```python
from build123d import *

# Parameters (mm, degrees)
F0_W      = 165
F0_H      = 45
F0_R      = 12.5
F1_DEPTH  = 1
F3_DEPTH  = 1
F4_DEPTH  = 25
F5_DEPTH  = 25
F8_DEPTH  = 1
F9_W      = 35.9933748841
F9_H      = 31.3726086169
F9_W_2    = 33.6829945445
F9_H_2    = 28.8190245628
F10_DEPTH = 1
F11_R     = 4.1249872097
F12_DEPTH = 25
F13_R     = 2.1502393586
F14_DEPTH = 25
F15_R     = 5
F16_DEPTH = 25


with BuildPart() as f1:
    # F0 (on Front) → F1 (new body)
    with BuildSketch(Plane.XZ):
        Rectangle(F0_W, F0_H)
        with Locations((-65, 0)):
            Circle(F0_R, mode=Mode.SUBTRACT)
        with Locations((65, 0)):
            Circle(F0_R, mode=Mode.SUBTRACT)
    extrude(amount=F1_DEPTH)

    # F2 (on face) → F3 (join)
    with BuildSketch(Plane.XZ.offset(1)):
        with BuildLine():
            Line((68.3925151825, -19.0988145769), (65, -22.5))
            ThreePointArc((65, -22.5), (87.5, 0), (65, 22.5))
            Line((65, 22.5), (71.474224329, 16.2770561874))
            Line((71.474224329, 16.2770561874), (77.4062722921, 9.1145541519))
            Line((77.4062722921, 9.1145541519), (80.3926512599, 2.1407562308))
            Line((80.3926512599, 2.1407562308), (80.3926512599, -5.2317115478))
            Line((80.3926512599, -5.2317115478), (78.3914923668, -12.1520543471))
            Line((78.3914923668, -12.1520543471), (74.6632069349, -14.4081749022))
            Line((74.6632069349, -14.4081749022), (68.3925151825, -19.0988145769))
        make_face()
        with BuildLine():
            Line((-65, 14.9617949501), (-65, 22.5))
            ThreePointArc((-65, 22.5), (-87.5, 0), (-65, -22.5))
            Line((-65, -22.5), (-67.4760043621, -15.6979020685))
            Line((-67.4760043621, -15.6979020685), (-72.8440880775, -12.9142012447))
            Line((-72.8440880775, -12.9142012447), (-76.5851810575, -7.8018400818))
            Line((-76.5851810575, -7.8018400818), (-79.5639529824, 0))
            Line((-79.5639529824, 0), (-79.5639529824, 6.4657721668))
            Line((-79.5639529824, 6.4657721668), (-75.4495188594, 11.7608513683))
            Line((-75.4495188594, 11.7608513683), (-65, 14.9617949501))
        make_face()
    extrude(amount=-F3_DEPTH)

    # F2 (on face) → F4 (cut)
    with BuildSketch(Plane.XZ.offset(1)):
        with BuildLine():
            Line((-82.5, 22.5), (-82.5, 14.1421356237))
            ThreePointArc((-82.5, 14.1421356237), (-74.6966991411, 20.3033008589), (-65, 22.5))
            Line((-65, 22.5), (-82.5, 22.5))
        make_face()
    extrude(amount=-F4_DEPTH, mode=Mode.SUBTRACT)

    # F2 (on face) → F5 (cut)
    with BuildSketch(Plane.XZ.offset(1)):
        with BuildLine():
            ThreePointArc((82.5, -14.1421356237), (74.6966991411, -20.3033008589), (65, -22.5))
            Line((65, -22.5), (82.5, -22.5))
            Line((82.5, -22.5), (82.5, -14.1421356237))
        make_face()
        with BuildLine():
            ThreePointArc((65, 22.5), (74.6966991411, 20.3033008589), (82.5, 14.1421356237))
            Line((82.5, 14.1421356237), (82.5, 22.5))
            Line((82.5, 22.5), (65, 22.5))
        make_face()
        with BuildLine():
            Line((-82.5, -22.5), (-65, -22.5))
            ThreePointArc((-65, -22.5), (-74.6966991411, -20.3033008589), (-82.5, -14.1421356237))
            Line((-82.5, -14.1421356237), (-82.5, -22.5))
        make_face()
    extrude(amount=-F5_DEPTH, mode=Mode.SUBTRACT)

    # F7 (on face) → F8 (join)
    with BuildSketch(Plane.XZ.offset(1)):
        Polygon((-81.9395110011, 0), (-87.5, 0), (-87.5, -22.5), (-65, -22.5), (-65, -18.5897927731), (-73.3228996396, -16.0001199692), (-80.1934376359, -9.6208481118), align=None)
    extrude(amount=-F8_DEPTH)

    # F9 (on face) → F10 (join)
    with BuildSketch(Plane.XZ.offset(1)):
        with Locations((-60.8671866357, 0.5391770974)):
            Rectangle(F9_W, F9_H)
        with Locations((63.7112520635, 0.1135794446)):
            Rectangle(F9_W_2, F9_H_2)
    extrude(amount=-F10_DEPTH)

    # F11 (on face) → F12 (cut)
    with BuildSketch(Plane.XZ.offset(1)):
        with Locations((65.292224288, 0)):
            Circle(F11_R)
    extrude(amount=-F12_DEPTH, mode=Mode.SUBTRACT)

    # F13 (on face) → F14 (cut)
    with BuildSketch(Plane.XZ.offset(1)):
        with Locations((-64.8811534047, 0)):
            Circle(F13_R)
    extrude(amount=-F14_DEPTH, mode=Mode.SUBTRACT)

    # F15 (on face) → F16 (cut)
    with BuildSketch(Plane(origin=(0, 0, 0), x_dir=(-1, 0, 0), z_dir=(0, 1, 0))):
        with Locations((-65.292224288, 0)):
            Circle(F15_R)
    extrude(amount=-F16_DEPTH, mode=Mode.SUBTRACT)


solid = f1.part
```
Part model, mm, in its own coordinate system. Round coordinates to 2 decimals unless told otherwise and drop trailing zeros. Write each loop counter-clockwise with the first axis right and the second up, starting at its lowest first coordinate (ties: lowest second). Pieces come first, ordered by that corner, then holes. Notation, with made-up numbers: (84.5, 20.5) -> (106.5, 20.5) arc R19 cw to (106.5, 49.5) -> close; hole circle Ø9 at (69, 52). An arc over 180 degrees is marked (long way). Return JSON: item names as keys, results as strings. Group by question number.
Q1. Saw through at B-B on z = -12. Write the cut outline in (x, y), plus the area to 3 significant figures.
Q2. Saw through at A-A on y = -0.8. Write the cut outline in (x, z).
Q3. Pin check, flat tip, straight feed: pin 1 (11.5 mm diameter, centred on x = 65.29, z = 0, fed in from +Y). Stop position of the tip, or through.
Q4. Probe L1, parallel to Z at x = -63, y = -0.05; L2, parallel to Z at x = -64, y = -0.05; L3, parallel to X at y = -0.9, z = 6.5. List the from-to ranges inside material, lowest first. Write a range as [from, to].
Q5. Mould opens along Z. For faces 1 (the flat face through (-1, -1, 0)), 2 (the cylindrical face through (-67.03, -0.51, 0.09)) say: pulls with the +Z half, pulls with the -Z half, needs draft (parallel to the pull), parting line crosses it, or undercut.
Answer:
{
 "1": {"outline": "(-87.5, -1) -> (84.03, -1) -> (84.03, 0) -> (-87.5, 0) -> close", "area": "172 mm2"},
 "2": {"outline": "(-87.5, -22.5) -> (65, -22.5) arc R22.5 ccw to (65, 22.5) -> (-65, 22.5) arc R22.5 ccw to (-87.5, 0) -> close; hole circle Ø4.3 at (-64.88, 0); hole circle Ø10 at (65.29, 0)"},
 "3": {"pin 1": "y = 0"},
 "4": {"L1": "[-22.5, -1.04], [1.04, 22.5]", "L2": "[-22.5, -1.96], [1.96, 22.5]", "L3": "[-86.54, 86.54]"},
 "5": {"face 1": "needs draft", "face 2": "undercut"}
}
